Autodesk Inventor part; units mm, degrees
ref_plane "YZ Plane" through (0, 0, 0) normal (1, 0, 0) x (0, 1, 0)
ref_plane "XZ Plane" through (0, 0, 0) normal (0, 1, 0) x (-1, 0, 0)
ref_plane "XY Plane" through (0, 0, 0) normal (0, 0, 1) x (1, 0, 0)
sketch "Sketch1" plane through (0, 0, 0) normal (0, 0, 1) x (1, 0, 0)
  line L0 (-490, 72) -> (490, 72)
  line L1 (490, 72) -> (490, 0)
  line L2 (490, 0) -> (-490, 0)
  line L3 (-490, 0) -> (-490, 72)
  point P0 (0, 0)
  point P1 (0, 0)
  dimension "d0" = 980
  dimension "d1" = 72
extrude "Plate1" add sketch "Sketch1" along normal blind 2
sketch "Sketch2" plane through (490, 2, 0) normal (0, -1, 0) x (1, 0, 0)
  line L0 (-980, 0) -> (0, 0)
  line L1 (0, 0) -> (0, 20)
  line L2 (0, 20) -> (-980, 20)
  line L3 (-980, 20) -> (-980, 0)
edge flange "Flange1" height 20 angle 90 thickness 2 bend radius 2.75 thickness toward (0, -1, 0) relief round relief width 2 relief depth 1 edges at (0, 0, 2) wall of the first edge with corners at (-490, 2, 0) (490, 2, 0) (490, 2, 20) (-490, 2, 20)
bend "Bend1"
corner "Corner1"
sketch "Sketch5" plane through (0, 0, 0) normal (0, 0, -1) x (-1, 0, 0)
  line L0 (490, 72) -> (-490, 72)
  line L1 (490, 0) -> (-490, 0)
  circle A0 centre (0, 72) radius 35
  line L2 (243.95, 72) -> (246.05, 72)
  line L3 (246.05, 72) -> (246.05, 27)
  line L4 (246.05, 27) -> (243.95, 27)
  line L5 (243.95, 27) -> (243.95, 72)
  line L6 (-243.95, 72) -> (-246.05, 72)
  line L7 (-246.05, 72) -> (-246.05, 27)
  line L8 (-246.05, 27) -> (-243.95, 27)
  line L9 (-243.95, 27) -> (-243.95, 72)
  line L10 (0, 72) -> (0, 0) construction
  line L11 (-490, 0) -> (-490, 72)
  line L12 (490, 0) -> (490, 72)
  circle A1 centre (-490, 72) radius 35
  circle A2 centre (490, 72) radius 35
  point P0 (0, 0)
  point P1 (245, 27)
  point P2 (-245, 27)
  point P3 (246.05, 72)
  point P4 (-35, 72)
  point P5 (35, 72)
  point P6 (-246.05, 72)
  point P7 (455, 72)
  point P8 (490, 37)
  point P9 (-490, 37)
  point P10 (-455, 72)
  dimension "d45" = 70
  dimension "d48" = 2.1
  dimension "d49" = 490
  dimension "d51" = 27
  dimension "d52" = 45
extrude "Extrusion1" cut sketch "Sketch5" against normal through all contours L3 L4 L5 L0 | L0 L12 A2 | L9 L8 L7 L0 | L11 L0 A1 picked at (487.4039, 48.9592) picked at (-466.9592, 69.4039)
sketch "Sketch9" plane through (0, 0, 2) normal (0, 0, 1) x (1, 0, 0)
  line L0 (-2.0322, 27.7998) -> (-2.0322, 15.7998) construction
  line L1 (-2.0322, 15.7998) -> (-202.0322, 15.7998) construction
  line L2 (-202.0322, 15.7998) -> (-202.0322, 27.7998) construction
  line L3 (-202.0322, 27.7998) -> (-2.0322, 27.7998) construction
  line L4 (-490, 72) -> (490, 72)
  point P0 (0, 0)
  point P1 (1.05, 68)
  point P2 (490, 72)
  point P3 (-490, 72)
  dimension "d40" = 200
  dimension "d41" = 12
mark "Mark2"
sketch "Sketch10" plane through (-243.95, 72, 2) normal (0, 0, 1) x (1, 0, 0)
  line L0 (-246.05, -72) -> (733.95, -72)
  line L1 (0, 0) -> (487.9, 0)
  line L2 (733.95, -72) -> (243.95, -72)
  line L3 (243.95, -72) -> (243.95, 0)
  line L4 (243.95, 0) -> (733.95, 0)
  line L5 (733.95, 0) -> (733.95, -72)
  point P0 (243.95, -72)
  point P1 (243.95, -72)
  dimension "d53" = 490
extrude "Extrusion4" cut sketch "Sketch10" along normal through all both and the other way through all
equation "\"d2\" = Thickness"
equation "\"d3\" = BendReliefWidth"
equation "\"d4\" = BendReliefDepth"
equation "\"d5\" = MinimumRemnant"
equation "\"d6\" = TransitionRadius"
equation "\"d9\" = BendRadius"
equation "\"d10\" = CornerReliefSize"
equation "\"d11\" = GapSize"
equation "\"d12\" = JacobiRadiusSize"
equation "\"BendReliefWidth\" = Thickness"
equation "\"BendReliefDepth\" = 0.5 * Thickness"
equation "\"CornerReliefSize\" = 4 * Thickness"
equation "\"MinimumRemnant\" = 2 * Thickness"
equation "\"TransitionRadius\" = BendRadius"
equation "\"JacobiRadiusSize\" = BendRadius"
equation "\"GapSize\" = Thickness"
properties part number "MSC 321 STRINGER BOARD  ####" material "Stainless Steel"
The model under review builds one solid part; all positions refer to its coordinate system, in mm. A direction names the side the tool comes from. Give positions to 0.01 mm unless a question says otherwise; leave off trailing zeros. Loops run counter-clockwise (first coordinate to the right, second up) from the corner with the lowest first, then second, coordinate; pieces in that order, holes last. Notation, with made-up numbers: (-21.5, -33) - (-8.5, -33) arc R17 cw to (-8.5, -1) - close; hole circle Ø10 at (74, 29.5). An arc over 180 degrees is marked (long way). Answer as a JSON object with one key per item and string values.
Q1. Add section B-B on x = -146. State the section outline as (y, z) points.
Worked out:
{"outline": "(0, 4.75) arc R4.75 ccw to (4.75, 0) - (72, 0) - (72, 2) - (4.75, 2) arc R2.75 cw to (2, 4.75) - (2, 20) - (0, 20) - close"}
Q2. For faces 1 (the flat face through (0, 27.8, 1.8)), 2 (the flat face through (-242, 2, 12)), list the 3-axis set-ups (+Z, -Z, +X, -X, +Y, -Y) from which the entire face can be reached by the end or side of a thin tool; tool diameter is ignored.
Worked out:
{"face 1": "+Z, -Z, +X, +Y, -Y", "face 2": "+Z, +X, -X, +Y"}
Q3. Add section A-A on y = 57. State the section outline as (x, z) points.
Worked out:
{"outline": "(-458.38, 0) - (-246.05, 0) - (-246.05, 2) - (-458.38, 2) - close; (-243.95, 0) - (0, 0) - (0, 2) - (-243.95, 2) - close"}
Q4. To check wall thickness, follow line 1 along Z through (x, y) = (-271, 28); line 2 along X through (y, z) = (60, 1). State the ranges of each line that lie inside material, in increasing order.
Worked out:
{"line 1": "z = 0 to 2", "line 2": "x = -457.12 to -246.05, -243.95 to 0"}
Q5. Insertion check: pin 1 (12 mm diameter, centred on x = -334, z = 12.5, fed in from +Y); pin 2 (1.6 mm diameter, centred on y = 41, z = 1, fed in from -X). Each pin has a flat end and moves straight along its axis. Give the tip position at first contact, or say it passes through.
Worked out:
{"pin 1": "stops at y = 2", "pin 2": "stops at x = -475.38"}
Q6. Add section C-C on z = 10.5. State the section outline as (x, y) points.
Worked out:
{"outline": "(-490, 0) - (0, 0) - (0, 2) - (-490, 2) - close"}
